Answer from the drawing. Dimensions are ordinates in mm from the lowest x, y and z of the part. A direction names the side the tool comes from. Round coordinates to 2 decimals unless told otherwise and drop trailing zeros. Order: outer loops, then holes, each group sorted by start corner. A loop starts at its lowest first (then second) coordinate and runs counter-clockwise, first axis right, second up.
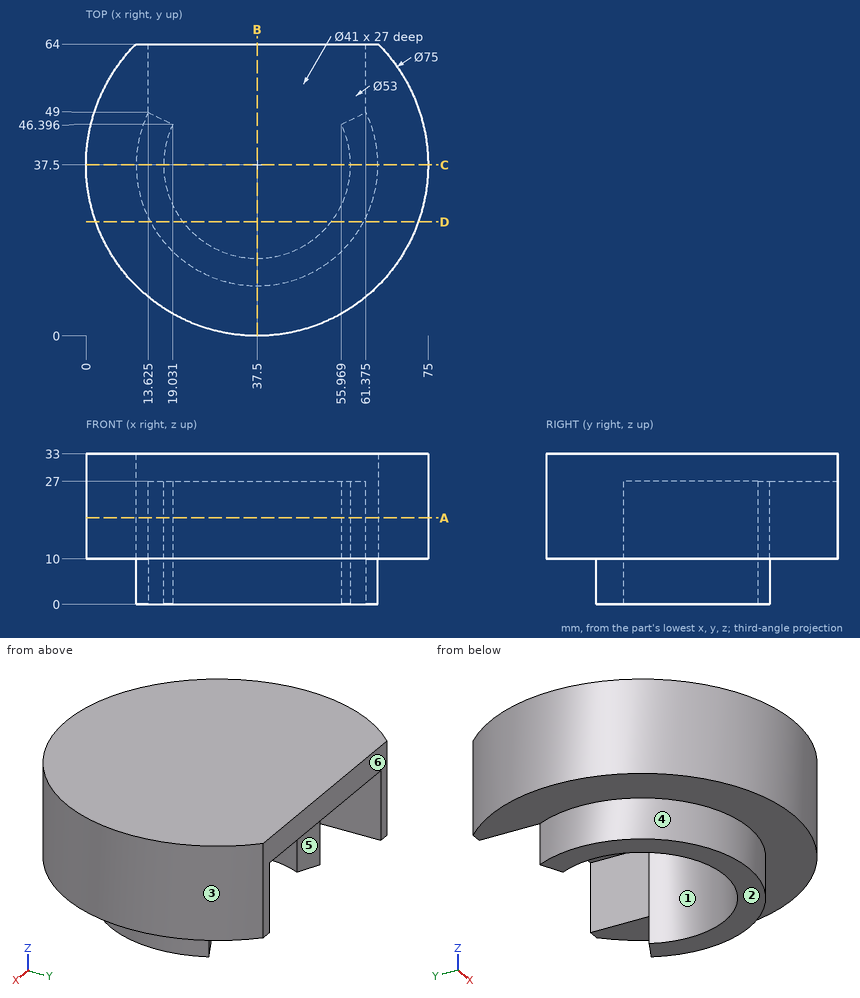
Q1. A cutting plane is placed at B-B, the plane x = 37.5. Give the vertices of the cut face in (y, z).
Outcome:
outline: (0, 10) - (11, 10) - (11, 0) - (17, 0) - (17, 27) - (64, 27) - (64, 33) - (0, 33) - close
Q2. Flat-ended cylindrical pins translate along their axes: pin 1 (12 mm diameter, centred on y = 55.5, z = 21, fed in from -X); pin 2 (16.5 mm diameter, centred on y = 53, z = 16.5, fed in from +X); pin 3 (8 mm diameter, centred on y = 34.5, z = 20, fed in from +X); pin 4 (1.5 mm diameter, centred on y = 48, z = 11.5, fed in from +X). Find the tip coordinate at first contact, or state that the pin passes through.
Outcome:
pin 1: stops at x = 1.97
pin 2: stops at x = 74.29
pin 3: stops at x = 75
pin 4: stops at x = 73.71
Q3. A cutting plane is placed at A-A, the plane z = 19. Give the vertices of the cut face in (x, y) (1 decimal), plus the area to 3 significant figures.
Outcome:
outline: (11, 64) arc R37.5 ccw (long way) to (64, 64) - (61.4, 64) - (61.4, 49) - (56, 46.4) arc R20.5 cw (long way) to (19, 46.4) - (13.6, 49) - (13.6, 64) - close
area: 2,180 mm2
Q4. A cutting plane is placed at C-C, the plane y = 37.5. Give the vertices of the cut face in (x, z), plus the area to 3 significant figures.
Outcome:
outline: (0, 10) - (11, 10) - (11, 0) - (17, 0) - (17, 27) - (58, 27) - (58, 0) - (64, 0) - (64, 10) - (75, 10) - (75, 33) - (0, 33) - close
area: 1,150 mm2
Q5. For a pull along X with two mould halves and no side action, classify the marked faces 1, 2 and 3 as released by +X, released by -X, zero draft, split by the parting line, or undercut.
Outcome:
face 1: undercut
face 2: zero draft
face 3: split by the parting line
Q6. Straight lines are drawn through the part: probe 1 along X at (y, z) = (37.5, 12.5); probe 2 along X at (y, z) = (37.5, 7.5); probe 3 along Z at (x, y) = (6.5, 17). For each, find the intervals that lie inside material, in ascending order.
Outcome:
probe 1: x = 0 to 17, 58 to 75
probe 2: x = 11 to 17, 58 to 64
probe 3: z = 10 to 33
Q7. For the marked faces 4, 5 and 6, determine the directions among +Z, -Z, +X, -X, +Y, -Y from which every point of the face is accessible in a straight line to the end or side of a thin tool.
Outcome:
face 4: -Z
face 5: -Z, +Y
face 6: +Z, -Z, +X, -X, +Y
Q8. A cutting plane is placed at D-D, the plane y = 25. Give the vertices of the cut face in (x, z) (1 decimal), plus the area to 3 significant figures.
Outcome:
outline: (2.1, 10) - (14.1, 10) - (14.1, 0) - (21.3, 0) - (21.3, 27) - (53.7, 27) - (53.7, 0) - (60.9, 0) - (60.9, 10) - (72.9, 10) - (72.9, 33) - (2.1, 33) - close
area: 1,220 mm2
